Part print with two shaded views. Sizes in mm from the minimum x, y, z corner. A direction names the side the tool comes from. Round coordinates to 2 decimals unless told otherwise and drop trailing zeros. Loops run counter-clockwise (first coordinate to the right, second up) from the corner with the lowest first, then second, coordinate; pieces in that order, holes last. Notation, with made-up numbers: (28.25, 5.25) - (43.25, 5.25) arc R32 ccw to (43.25, 43.25) - close; hole circle Ø7 at (29, 40). An arc over 180 degrees is marked (long way). Use a Markdown table: item, result.
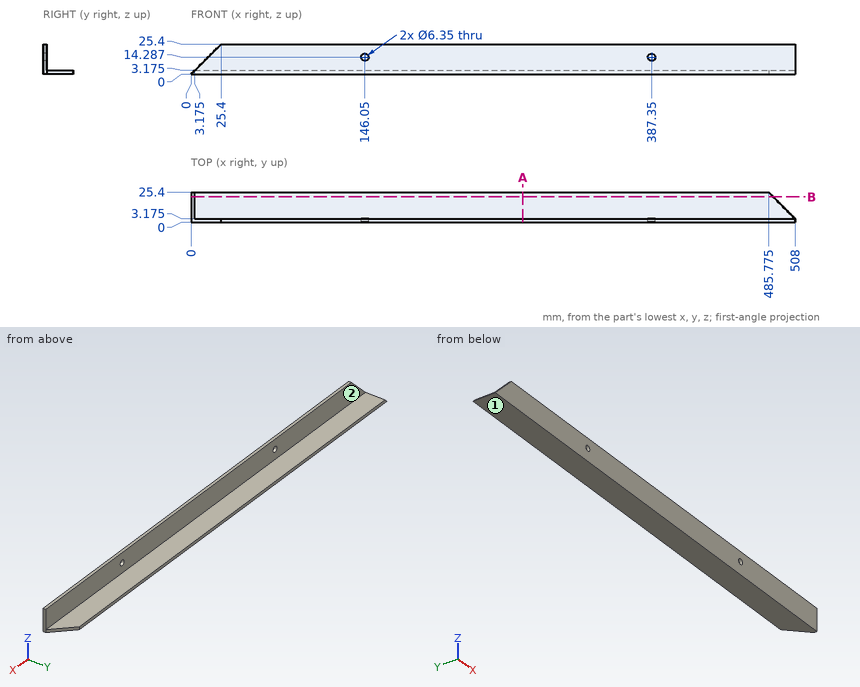
Q1. Cut at B-B, the plane y = 21.5. List the corners of the cut face in (x, z) (1 decimal), plus the area to 3 significant figures.
Results found:
| item | result |
|---|---|
| outline | (0, 0) - (489.7, 0) - (489.7, 3.2) - (3.2, 3.2) - close |
| area | 1,550 mm2 |
Q2. Cut at A-A, the plane x = 279. List the corners of the cut face in (y, z) (1 decimal), plus the area to 3 significant figures.
Results found:
| item | result |
|---|---|
| outline | (0, 0) - (25.4, 0) - (25.4, 3.2) - (3.2, 3.2) - (3.2, 25.4) - (0, 25.4) - close |
| area | 151 mm2 |
Q3. Probe line 1 (Z direction, x = 387.35, y = 1.8); line 2 (Y direction, x = 243.5, z = 9.5) (1 decimal). List the from-to ranges inside material, lowest first.
Results found:
| item | result |
|---|---|
| line 1 | z = 0 to 11.11, 17.46 to 25.4 |
| line 2 | y = 0 to 3.2 |
Q4. Drop flat-ended pins along their axis: pin 1 (1.5 mm diameter, centred on x = 398, y = 11.5, fed in from +Z) (1 decimal); pin 2 (4 mm diameter, centred on x = 387.35, z = 14.29, fed in from -Y); pin 3 (1.5 mm diameter, centred on x = 378, z = 14.5, fed in from +Y) (1 decimal). Give the stop position or say it passes through.
Results found:
| item | result |
|---|---|
| pin 1 | stops at z = 3.2 |
| pin 2 | passes through |
| pin 3 | stops at y = 3.2 |
Q5. Which spindle directions (+Z, -Z, +X, -X, +Y, -Y) get a long thin tool onto all of the face, cutting with end or side? Do the marked faces 1 and 2. Say none if no direction does.
Results found:
| item | result |
|---|---|
| face 1 | -Z, +X, -X, +Y, -Y |
| face 2 | +Z, +X, -X, +Y |
